Input: part model. Units: mm. Frame: model coordinates. A direction names the side the tool comes from. Coordinates: 2 decimals unless noted, no trailing zeros. Write each loop counter-clockwise with the first axis right and the second up, starting at its lowest first coordinate (ties: lowest second). Pieces come first, ordered by that corner, then holes. Notation, with made-up numbers: (73, -33.5) - (130, -33.5) arc R23 ccw to (130, -16.5) - close; hole circle Ø2 at (67.25, 57). An arc over 180 degrees is marked (long way). Use a Markdown table: item, result. Add a question column.
Q1. Material intervals for probe 1 along X at (y, z) = (-26, -28); probe 2 along Z at (x, y) = (6.5, 0.5); probe 3 along Z at (x, y) = (17.5, -13.5), sorted ascending. Write a range as from..to.
Q2. Section query A-A (x = 0). Return the cut outline in (y, z), then the cut area to 3 significant figures.
Q3. Pin query (flat end, axial travel): P1, Ø5, axis at x = 9.5, z = -17.5, coming from the +Y side; P2, Ø6, axis at x = 0.5, z = 24, coming from the +Y side; P3, Ø10, axis at x = 3.5, z = 28.5, coming from the +Y side; P4, Ø16, axis at x = -4.5, z = -2.5, coming from the -Y side. Return the tip coordinate at first contact, or that it passes through.
Q4. Mould query, pull axis Y, two halves, no side actions, for faces 6 (the face through (19.31, -20.36, -34.04)), 7 (the face through (-0.716, -23.289, -5.453)), 8 (the face through (-9, -33, 5)). Classes: released by +Y, released by -Y, zero draft, split by the parting line, or undercut.
Q5. Section query B-B (y = -24.5). Return the cut outline in (x, z).
Q6. Set-up query: faces 1 (the face through (-16.2, -20.1, -34.5)), 2 (the face through (-19.39, -23.92, 21.42)), 3 (the face through (-0.88, -27.88, 19.98)), 4 (the face through (-2.87, 30.03, 6.93)), 5 (the face through (19.39, -23.92, 21.42)). Return all of +Z, -Z, +X, -X, +Y, -Y with unobstructed straight access to the full face (end or side cutting, diameter ignored); none if empty.
Q7. Section query C-C (z = 0). Give the number of separate pieces and of enclosed holes in the cut face, then the cut area to 3 significant figures.
Q8. Section query D-D (y = -7.5). Return the cut outline in (x, z).
from build123d import *
from build123d.topology import SkipClean

# Parameters (mm, degrees)
SKETCH1_R                = 28
SKETCH1_R_2              = 19.5
BOSS_EXTRUDE1_DEPTH      = 22.5
BOSS_EXTRUDE2_REACH      = 72.79
BOSS_EXTRUDE2_END_RADIUS = 28
SKETCH2_R                = 7.5
BOSS_EXTRUDE3_REACH      = 77.142
BOSS_EXTRUDE3_END_RADIUS = 28
SKETCH3_R                = 20
HOLE1_D                  = 11
HOLE1_CBORE_D            = 20
HOLE1_CBORE_DEPTH        = 5
BOSS_EXTRUDE4_DEPTH      = 6.3
CIRPATTERN2_COUNT        = 3
MIRROR3_COPY_1_DEPTH     = 6.3
MIRROR3_COPY_2_DEPTH     = 6.3
HOLE4_D                  = 9.4
HOLE4_DEPTH              = 6.3
HOLE5_D                  = 9.4
HOLE5_DEPTH              = 6.3


with BuildPart() as part:
    # Sketch1 → Boss-Extrude1 (new, symmetric)
    with BuildSketch(Plane(origin=(0, 0, 0), x_dir=(0, 0, -1), z_dir=(1, 0, 0))):
        with Locations(Location((0, 0, 0), (0, 0, 180))):
            Circle(SKETCH1_R)
        with Locations(Location((0, 0, 0), (0, 0, 180))):
            Circle(SKETCH1_R_2, mode=Mode.SUBTRACT)
    extrude(amount=BOSS_EXTRUDE1_DEPTH, both=True)

    # Boss-Extrude2: up to this cylinder (the profile starts outside it)
    boss_extrude2_end = Plane(origin=(0, 0, 0), z_dir=(-1, 0, 0)) * Cylinder(BOSS_EXTRUDE2_END_RADIUS, 202.58, mode=Mode.PRIVATE)
    # Sketch2 → Boss-Extrude2 (add, up to the surface)
    with BuildSketch(Plane(origin=(0, 33, 0), x_dir=(1, 0, 0), z_dir=(0, 1, 0)), mode=Mode.PRIVATE) as boss_extrude2_sk1:
        with Locations(Location((0, 0, 0), (0, 0, 270))):
            Circle(SKETCH2_R)
    boss_extrude2_tool1 = extrude(boss_extrude2_sk1.sketch, amount=-BOSS_EXTRUDE2_REACH, mode=Mode.PRIVATE) - boss_extrude2_end
    add(boss_extrude2_tool1.solids().sort_by_distance((0, 33, 0))[0])

    # Boss-Extrude3: up to this cylinder (the profile starts outside it)
    boss_extrude3_end = Plane(origin=(0, 0, 0), z_dir=(-1, 0, 0)) * Cylinder(BOSS_EXTRUDE3_END_RADIUS, 211.284, mode=Mode.PRIVATE)
    # Sketch3 → Boss-Extrude3 (add, up to the surface)
    with BuildSketch(Plane(origin=(0, -33, 0), x_dir=(1, 0, 0), z_dir=(0, 1, 0)), mode=Mode.PRIVATE) as boss_extrude3_sk1:
        with Locations(Location((0, 0, 0), (0, 0, 90))):
            Circle(SKETCH3_R)
    boss_extrude3_tool1 = extrude(boss_extrude3_sk1.sketch, amount=BOSS_EXTRUDE3_REACH, mode=Mode.PRIVATE) - boss_extrude3_end
    add(boss_extrude3_tool1.solids().sort_by_distance((0, -33, 0))[0])

    # Hole1 (through all)
    with Locations(Plane(origin=(0, -33, 0), x_dir=(-1, 0, 0), z_dir=(0, -1, 0))):
        with Locations((0, 0)):
            CounterBoreHole(HOLE1_D / 2, HOLE1_CBORE_D / 2, HOLE1_CBORE_DEPTH)

    # Sketch6 → Boss-Extrude4 (add)
    with BuildSketch(Plane.ZY.offset(22.5)):
        with BuildLine():
            Line((-10.004005993, 35), (-10.004005993, 16.738275422))
            ThreePointArc((-10.004005993, 16.738275422), (0, 19.5), (10.004005993, 16.738275422))
            Line((10.004005993, 16.738275422), (10.004005993, 35))
            ThreePointArc((10.004005993, 35), (0, 45.004005993), (-10.004005993, 35))
        make_face()
    boss_extrude4 = extrude(amount=-BOSS_EXTRUDE4_DEPTH)

    # CirPattern2: Boss-Extrude4 ×3 about axis
    with SkipClean():  # the faces are left unmerged after this step: merging them gives an invalid solid
        cirpattern2_axis = Axis((0, 0, 0), (1, 0, 0))
        for i in range(1, CIRPATTERN2_COUNT):
            add(boss_extrude4.rotate(cirpattern2_axis, i * 360 / CIRPATTERN2_COUNT))

    # Mirror3: Boss-Extrude4 across plane
    add(boss_extrude4.mirror(Plane(origin=(0, 0, 0), x_dir=(0, 0, 1), z_dir=(1, 0, 0))))

    # Mirror3 copy 1 sketch → Mirror3 copy 1 (add)
    with SkipClean():  # the faces are left unmerged after this step: merging them gives an invalid solid
        with BuildSketch(Plane(origin=(22.5, 0, 0), x_dir=(0, -0.8660254037844387, -0.4999999999999998), z_dir=(1, 0, 0))):
            with BuildLine():
                Line((-10.004005993, -35), (-10.004005993, -16.738275422))
                ThreePointArc((-10.004005993, -16.738275422), (0, -19.5), (10.004005993, -16.738275422))
                Line((10.004005993, -16.738275422), (10.004005993, -35))
                ThreePointArc((10.004005993, -35), (0, -45.004005993), (-10.004005993, -35))
            make_face()
        extrude(amount=-MIRROR3_COPY_1_DEPTH)

    # Mirror3 copy 2 sketch → Mirror3 copy 2 (add)
    with SkipClean():  # the faces are left unmerged after this step: merging them gives an invalid solid
        with BuildSketch(Plane(origin=(22.5, 0, 0), x_dir=(0, 0.8660254037844384, -0.5000000000000004), z_dir=(1, 0, 0))):
            with BuildLine():
                Line((-10.004005993, -35), (-10.004005993, -16.738275422))
                ThreePointArc((-10.004005993, -16.738275422), (0, -19.5), (10.004005993, -16.738275422))
                Line((10.004005993, -16.738275422), (10.004005993, -35))
                ThreePointArc((10.004005993, -35), (0, -45.004005993), (-10.004005993, -35))
            make_face()
        extrude(amount=-MIRROR3_COPY_2_DEPTH)
    add(part.part.scale(1), mode=Mode.REPLACE)  # the faces are merged on a copy

    # Hole4
    with Locations(Plane.ZY.offset(22.5)):
        with Locations((30.310889132, -17.5), (0, 35), (-30.310889132, -17.5)):
            Hole(HOLE4_D / 2, depth=HOLE4_DEPTH)

    # Hole5
    with Locations(Plane(origin=(22.5, 0, 0), x_dir=(0, 0, -1), z_dir=(1, 0, 0))):
        with Locations((0, 35), (30.310889132, -17.5), (-30.310889132, -17.5)):
            Hole(HOLE5_D / 2, depth=HOLE5_DEPTH)


solid = part.part
Values follow:
| question | item | result |
|---|---|---|
| 1 | probe 1 | -22.5..-16.2, 16.2..22.5 |
| 1 | probe 2 | -28..-19.49, 19.49..28 |
| 1 | probe 3 | -39.48..-32.78, -27.84..-14.07, 14.07..27.84, 32.78..39.48 |
| 2 | outline | (-33, -20) - (-19.6, -20) arc R28 ccw to (26.98, -7.5) - (33, -7.5) - (33, -5.5) - (18.71, -5.5) arc R19.5 cw to (-18.71, -5.5) - (-28, -5.5) - (-28, -10) - (-33, -10) - close; (-33, 10) - (-28, 10) - (-28, 5.5) - (-18.71, 5.5) arc R19.5 cw to (18.71, 5.5) - (33, 5.5) - (33, 7.5) - (26.98, 7.5) arc R28 ccw to (-19.6, 20) - (-33, 20) - close |
| 2 | area | 1,310 mm2 |
| 3 | P1 | y = 23.64 |
| 3 | P2 | y = 18.52 |
| 3 | P3 | y = 15.22 |
| 3 | P4 | y = -33 |
| 4 | face 6 | undercut |
| 4 | face 7 | zero draft |
| 4 | face 8 | released by -Y |
| 5 | outline | (-22.5, -37.46) - (-16.2, -37.46) - (-16.2, -22.43) - (-22.5, -22.43) - close; (-22.5, -13.56) - (-14.71, -13.56) arc R20 ccw to (14.71, -13.56) - (22.5, -13.56) - (22.5, 13.56) - (14.71, 13.56) arc R20 ccw to (-14.71, 13.56) - (-22.5, 13.56) - close; (-22.5, 22.43) - (-16.2, 22.43) - (-16.2, 37.46) - (-22.5, 37.46) - close; (16.2, -37.46) - (22.5, -37.46) - (22.5, -22.43) - (16.2, -22.43) - close; (16.2, 22.43) - (22.5, 22.43) - (22.5, 37.46) - (16.2, 37.46) - close; hole circle Ø11 at (0, 0) |
| 6 | face 1 | -Z, -Y |
| 6 | face 2 | -X, -Y |
| 6 | face 3 | -Y |
| 6 | face 4 | +Y |
| 6 | face 5 | +X, -Y |
| 7 | separate pieces | 6 |
| 7 | enclosed holes | 0 |
| 7 | area | 794 mm2 |
| 8 | outline | (-22.5, -33) - (-16.2, -33) - (-16.2, -26.98) - (16.2, -26.98) - (16.2, -33) - (22.5, -33) - (22.5, -18) - (-22.5, -18) - close; (-22.5, 18) - (22.5, 18) - (22.5, 33) - (16.2, 33) - (16.2, 26.98) - (-16.2, 26.98) - (-16.2, 33) - (-22.5, 33) - close |
